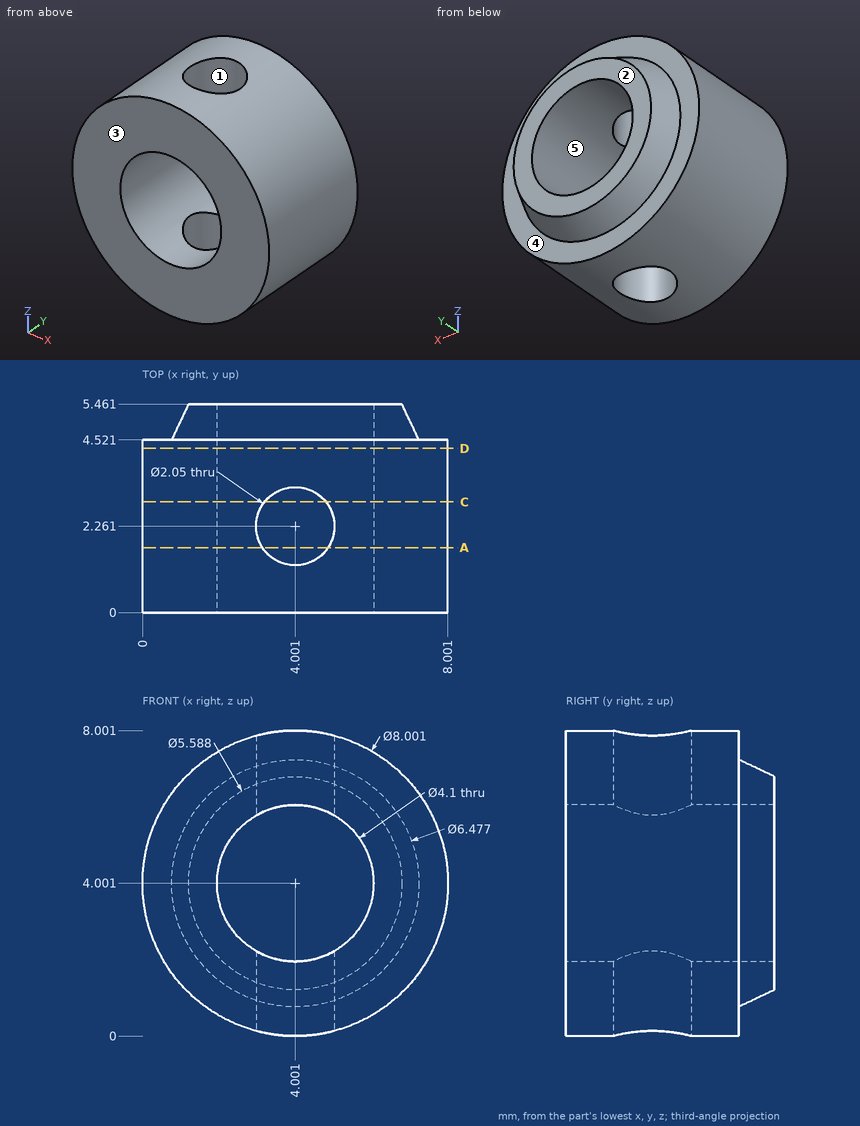
Job drawing, mm, ordinate dimensions from the low corner. One solid piece. A direction names the side the tool comes from. Coordinates: 2 decimals unless noted, no trailing zeros. Order: outer loops, then holes, each group sorted by start corner. A loop starts at its lowest first (then second) coordinate and runs counter-clockwise, first axis right, second up. Notation, with made-up numbers: (-30.75, 26.5) - (-26.75, 26.5) arc R6 ccw to (-26.75, 33.5) - close; hole circle Ø3 at (4.5, -28.5). An arc over 180 degrees is marked (long way). Use CSV: the item, a comma, the result in double quotes.
Item 1: Saw through at A-A on y = 1.7. Give the cut face in (x, z).
Solved:
outline,"(3.14, 0.09) - (3.14, 2.14) arc R2.05 cw to (3.14, 5.86) - (3.14, 7.91) arc R4 ccw to start; (4.86, 0.09) arc R4 ccw to (4.86, 7.91) - (4.86, 5.86) arc R2.05 cw to (4.86, 2.14) - close"
Item 2: Mould opens along Y. For the marked faces 1, 2 and 3 say: +Y half, -Y half, draft (parallel to the pull), parting line (faces both ways), or undercut.
Solved:
face 1,"undercut"
face 2,"+Y half"
face 3,"-Y half"
Item 3: Saw through at D-D on y = 4.3. Give the cut face in (x, z).
Solved:
outline,"circle Ø8 at (4, 4); hole circle Ø4.1 at (4, 4)"
Item 4: Saw through at C-C on y = 2.9. Give the cut face in (x, z).
Solved:
outline,"(3.2, 0.08) - (3.2, 2.11) arc R2.05 cw to (3.2, 5.89) - (3.2, 7.92) arc R4 ccw to start; (4.8, 0.08) arc R4 ccw to (4.8, 7.92) - (4.8, 5.89) arc R2.05 cw to (4.8, 2.11) - close"
Item 5: Drop a flat-ended pin along its axis: P1, Ø1.5, axis at y = 1, z = 6, coming from the +X side. Give the stop position or say it passes through.
Solved:
P1,"stops at x = 7.8"
Item 6: 3-axis set-ups, long thin cutter, end or side, ignore diameter. For the marked faces 4 and 5: which of +Z, -Z, +X, -X, +Y, -Y reach the whole face in a straight line?
Solved:
face 4,"+Y"
face 5,"+Y, -Y"
Item 7: Probe probe 1 along Y at (x, z) = (1.5, 6.5); probe 2 along Z at (x, y) = (4.5, 0.75); probe 3 along Z at (x, y) = (3, 0.2) (1 decimal). List the from-to ranges inside material, lowest first.
Solved:
probe 1,"y = 0 to 4.52"
probe 2,"z = 0.03 to 2.01, 5.99 to 7.97"
probe 3,"z = 0.1 to 2.2, 5.8 to 7.9"
